Can you work these out from the model? Positions are in its coordinate system, mm. Face numbers are marked on the shaded views. A direction names the side the tool comes from. Give positions to 0.01 mm unless a question says otherwise; leave off trailing zeros. Loops run counter-clockwise (first coordinate to the right, second up) from the corner with the lowest first, then second, coordinate; pieces in that order, holes last. Notation, with made-up numbers: M 12.5,57 L 45.5,57 A14 cw 45.5,76 Z; hole C 1,2 d5. An arc over 180 degrees is marked long. Use CSV: the item, a comma, the result in double quotes.
from build123d import *

# Parameters (mm, degrees)
BOSS_EXTRUDE1_DEPTH         = 15
TAP_DRILL_FOR_M3X0_5_TAP1_D = 2.5


with BuildPart() as part:
    # Sketch1 → Boss-Extrude1 (new body)
    with BuildSketch(Plane.XY):
        with BuildLine():
            Line((-30.590304709, 0), (-27.590304709, 0))
            ThreePointArc((-27.590304709, 0), (-18.390304709, 9.2), (-9.190304709, 0))
            Line((-9.190304709, 0), (-9.190304709, -9.2))
            Line((-9.190304709, -9.2), (-5.190304709, -9.2))
            Line((-5.190304709, -9.2), (-5.190304709, 0))
            ThreePointArc((-5.190304709, 0), (4.009695291, 9.2), (13.209695291, 0))
            Line((13.209695291, 0), (13.209695291, -9.2))
            Line((13.209695291, -9.2), (17.209695291, -9.2))
            Line((17.209695291, -9.2), (17.209695291, 0))
            ThreePointArc((17.209695291, 0), (26.409695291, 9.2), (35.609695291, 0))
            Line((35.609695291, 0), (38.609695291, 0))
            ThreePointArc((38.609695291, 0), (35.036398021, 8.62670273), (26.409695291, 12.2))
            Line((26.409695291, 12.2), (-18.390304709, 12.2))
            ThreePointArc((-18.390304709, 12.2), (-27.01700744, 8.62670273), (-30.590304709, 0))
        make_face()
    extrude(amount=BOSS_EXTRUDE1_DEPTH)

    # Tap Drill for M3x0.5 Tap1 (through all)
    with Locations(Plane(origin=(0, -9.2, 0), x_dir=(-1, 0, 0), z_dir=(0, -1, 0))):
        with Locations((7.190304709, -7.5), (-15.209695291, -7.5)):
            Hole(TAP_DRILL_FOR_M3X0_5_TAP1_D / 2)


solid = part.part
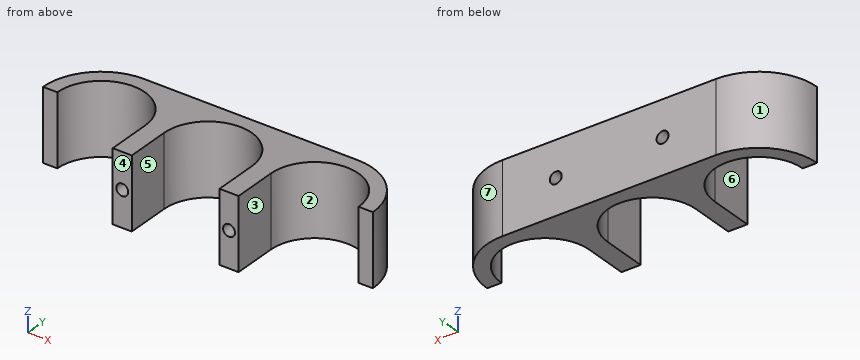
Q1. I'm going to push flat-ended pins straight in: P1, Ø4.5, axis at y = -6, z = 9.5, coming from the -X side; P2, Ø2.5, axis at x = 37, z = 11, coming from the -Y side; P3, Ø4, axis at x = 29, z = 2, coming from the -Y side; P4, Ø6, axis at x = 9, y = 1, coming from the -Z side. Where does each tip first touch, or does it pass through?
Model answer:
P1,"x = -9.19"
P2,"y = 0"
P3,"y = 7.97"
P4,"through"
Q2. I want a section at B-B, the plane z = 7.5. Please give me the cut outline in (x, y), then the cut area to 3 significant figures.
Model answer:
outline,"M -30.59,0 L -27.59,0 A9.2 cw -9.19,0 L -9.19,-9.2 L -8.44,-9.2 L -8.44,12.2 L -18.39,12.2 A12.2 ccw Z; M -5.94,-9.2 L -5.19,-9.2 L -5.19,0 A9.2 cw 13.21,0 L 13.21,-9.2 L 13.96,-9.2 L 13.96,12.2 L -5.94,12.2 Z; M 16.46,-9.2 L 17.21,-9.2 L 17.21,0 A9.2 cw 35.61,0 L 38.61,0 A12.2 ccw 26.41,12.2 L 16.46,12.2 Z"
area,"348 mm2"
Q3. Please list where these lines run through material, in increasing order: L1, parallel to X at y = -3.5, z = 7.5; L2, parallel to X at y = 3, z = 12.25; L3, parallel to X at y = 3, z = 7.5. Write a range as from..to.
Model answer:
L1,"-9.19..-8.44, -5.94..-5.19, 13.21..13.96, 16.46..17.21"
L2,"-30.22..-27.09, -9.69..-4.69, 12.71..17.71, 35.11..38.24"
L3,"-30.22..-27.09, -9.69..-8.44, -5.94..-4.69, 12.71..13.96, 16.46..17.71, 35.11..38.24"
Q4. I want a section at D-D, the plane z = 1.25. Please give me the cut outline in (x, y), then the cut area to 3 significant figures.
Model answer:
outline,"M -30.59,0 L -27.59,0 A9.2 cw -9.19,0 L -9.19,-9.2 L -5.19,-9.2 L -5.19,0 A9.2 cw 13.21,0 L 13.21,-9.2 L 17.21,-9.2 L 17.21,0 A9.2 cw 35.61,0 L 38.61,0 A12.2 ccw 26.41,12.2 L -18.39,12.2 A12.2 ccw Z"
area,"455 mm2"
Q5. I want a section at A-A, the plane y = -2. Please give me the cut outline in (x, z).
Model answer:
outline,"M -9.19,0 L -5.19,0 L -5.19,15 L -9.19,15 Z; M 13.21,0 L 17.21,0 L 17.21,15 L 13.21,15 Z; hole C -7.19,7.5 d2.5; hole C 15.21,7.5 d2.5"
Q6. If we mould it in two halves opening along X, with no side actions, what happens to the marked faces 1, 2, 3 and 4? For each: released by +X, released by -X, zero draft, split by the parting line, or undercut.
Model answer:
face 1,"released by -X"
face 2,"undercut"
face 3,"released by +X"
face 4,"zero draft"
Q7. I want a section at C-C, the plane y = 8. Please give me the cut outline in (x, z), then the cut area to 3 significant figures.
Model answer:
outline,"M -27.6,0 L -22.93,0 L -22.93,15 L -27.6,15 Z; M -13.85,0 L -0.53,0 L -0.53,15 L -13.85,15 Z; M 8.55,0 L 21.87,0 L 21.87,15 L 8.55,15 Z; M 30.95,0 L 35.62,0 L 35.62,15 L 30.95,15 Z; hole C -7.19,7.5 d2.5; hole C 15.21,7.5 d2.5"
area,"530 mm2"
Q8. For the marked faces 5, 6 and 7, which set-ups out of +Z, -Z, +X, -X, +Y, -Y let a thin tool reach every point of the face, with its end or its side?
Model answer:
face 5,"+Z, -Z, -Y"
face 6,"+Z, -Z, -X, -Y"
face 7,"+Z, -Z, +X, +Y"
